For this review, use the dimensioned drawing (mm, ordinates from the lowest corner) and the shaded views. A direction names the side the tool comes from. Coordinates: 2 decimals unless noted, no trailing zeros. Loops run counter-clockwise (first coordinate to the right, second up) from the corner with the lowest first, then second, coordinate; pieces in that order, holes last. Notation, with made-up numbers: (10, 11) -> (51, 11) arc R18 cw to (51, 32) -> close; hole circle Ø2 at (76.25, 51). An arc over 180 degrees is marked (long way). One line per question, with ' | ' between items. Start each with the question number.
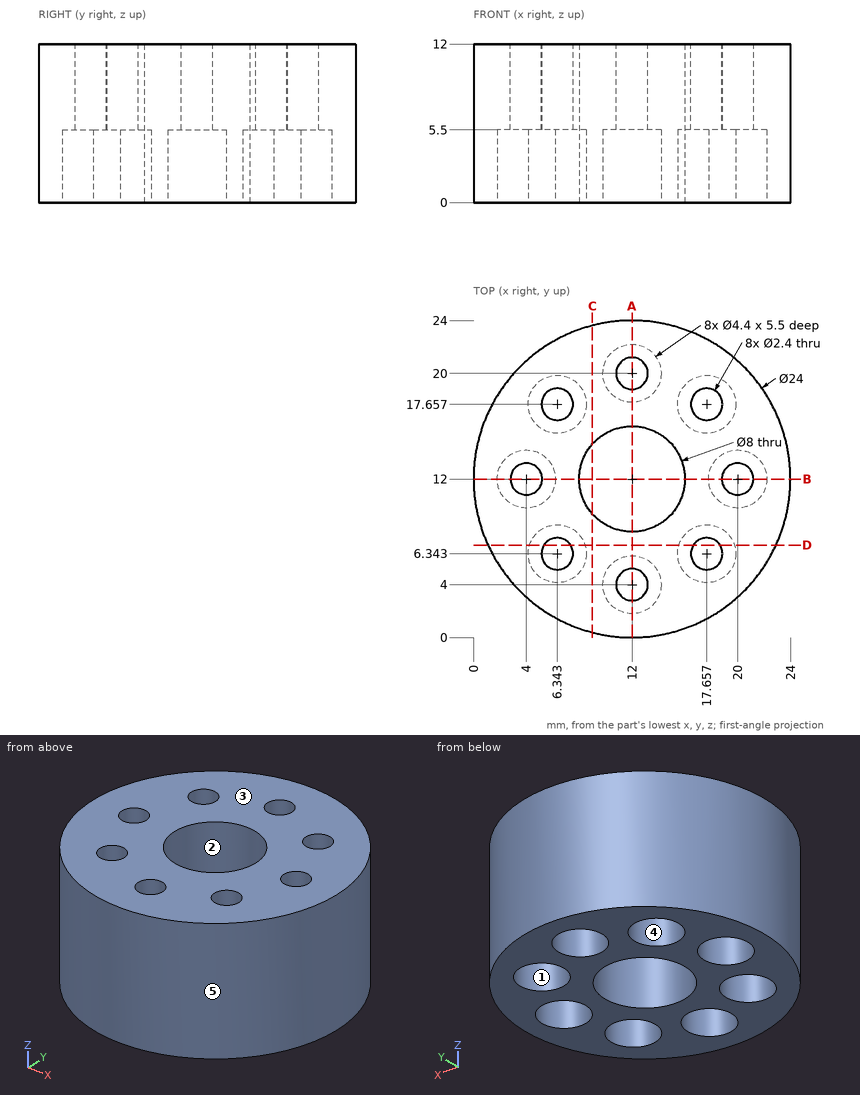
1) Consider section A-A, the plane x = 12. Write out the cut boundary in (y, z).
2) Wall thickness on L1, parallel to Y at x = 12, z = 4.25; L2, parallel to Y at x = 18.5, z = 10; L3, parallel to X at y = 11.75, z = 8.25: over which ranges is each line inside the solid? List them lowest first.
3) Consider section D-D, the plane y = 7. Write out the cut boundary in (x, z), plus the area to 4 significant figures.
4) Mouldability with a two-part tool opening along Y and no side actions: class the marked faces 3, 4 and 5 as +Y half, -Y half, draft (parallel to the pull), parting line (faces both ways), or undercut.
5) Consider section C-C, the plane x = 9. Write out the cut boundary in (y, z), plus the area to 3 significant figures.
6) Insertion check: pin 1 Ø3 at (x, z) = (21.5, 4) entering from -Y; pin 2 Ø1.9 at (x, y) = (4, 12) entering from -Z; pin 3 Ø2 at (x, y) = (12.5, 21) entering from -Z; pin 4 Ø6 at (x, z) = (5, 10) entering from -Y. Each pin has a flat end and moves straight along its axis. Give the tip position at first contact, or say it passes through.
7) Machinability: for the marked faces 1 and 2, which of the approach directions +Z, -Z, +X, -X, +Y, -Y give a long, thin tool a straight path to every point of the face, cutting with its end or side? Answer none if there is none.
Filled sheet:
1) outline: (0, 0) -> (1.8, 0) -> (1.8, 5.5) -> (2.8, 5.5) -> (2.8, 12) -> (0, 12) -> close; (5.2, 5.5) -> (6.2, 5.5) -> (6.2, 0) -> (8, 0) -> (8, 12) -> (5.2, 12) -> close; (16, 0) -> (17.8, 0) -> (17.8, 5.5) -> (18.8, 5.5) -> (18.8, 12) -> (16, 12) -> close; (21.2, 5.5) -> (22.2, 5.5) -> (22.2, 0) -> (24, 0) -> (24, 12) -> (21.2, 12) -> close
2) L1: 0 to 1.8, 6.2 to 8, 16 to 17.8, 22.2 to 24 | L2: 1.91 to 5.49, 7.2 to 16.8, 18.51 to 22.09 | L3: 0 to 2.83, 5.17 to 8.01, 15.99 to 18.83, 21.17 to 24
3) outline: (1.09, 0) -> (4.24, 0) -> (4.24, 5.5) -> (5.34, 5.5) -> (5.34, 12) -> (1.09, 12) -> close; (7.35, 5.5) -> (8.44, 5.5) -> (8.44, 0) -> (15.56, 0) -> (15.56, 5.5) -> (16.65, 5.5) -> (16.65, 12) -> (7.35, 12) -> close; (18.66, 5.5) -> (19.76, 5.5) -> (19.76, 0) -> (22.91, 0) -> (22.91, 12) -> (18.66, 12) -> close | area: 189.5 mm^2
4) face 3: draft | face 4: undercut | face 5: parting line
5) outline: (0.38, 0) -> (9.35, 0) -> (9.35, 12) -> (0.38, 12) -> close; (14.65, 0) -> (23.62, 0) -> (23.62, 12) -> (14.65, 12) -> close | area: 215 mm^2
6) pin 1: y = 3.06 | pin 2: through | pin 3: z = 5.5 | pin 4: y = 0.69
7) face 1: -Z | face 2: +Z, -Z
